Geometry: final body of the model. Coordinates: model frame, mm. A direction names the side the tool comes from. Give positions to 0.01 mm unless a question says otherwise; leave off trailing zeros. Write each loop counter-clockwise with the first axis right and the second up, starting at its lowest first coordinate (ties: lowest second). Pieces come first, ordered by that corner, then holes.
Q1. Cut plane B-B on y = -2.3. Return the cut outline in (x, z), plus the area to 3 significant figures.
Q2. Reachability of faces 5 (the face through (2.848, 0, 12)), 6 (the face through (-2.6, 0.7, 11)) from +Z, -Z, +X, -X, +Y, -Y: full face, straight path, thin tool, end or side. Return the list, or none.
Q3. Pin query (flat end, axial travel): pin 1 (3 mm diameter, centred on x = 0.5, y = 0, fed in from -Z) (3 decimals). Return the tip coordinate at first contact, or that it passes through.
Q4. Draft query along Y for faces 1 (the face through (0, -2.79, 12)), 2 (the face through (0.1, -0.3, 10.9)), 3 (the face through (-1.216, 1.115, 5.306)), 4 (the face through (-0.54, -2.44, 5.42)). Return one class per face: pulls with the +Y half, pulls with the -Y half, needs draft (parallel to the pull), parting line crosses it, or undercut.
Q5. Cut plane A-A on z = 1.75. Return the cut outline in (x, y).
Q6. Line query: L1, parallel to Y at x = 0, z = 6.25; L2, parallel to Y at x = -1.35, z = 7; L3, parallel to Z at x = -2.55, y = 1.05. Output: solid intervals per line, ascending.
```python
from build123d import *

# Parameters (mm, degrees)
SKETCH_1_R                   = 2.5
EXTRUDE_1_DEPTH              = 11
SKETCH_2_W                   = 5.696018396
SKETCH_2_H                   = 5.580245664
EXTRUDE_2_DEPTH              = 2
HOLE_WIZARD_M4_1_D           = 3.3
HOLE_WIZARD_M4_1_DEPTH       = 10.1
HOLE_WIZARD_M4_1_CSINK_D     = 4.05
HOLE_WIZARD_M4_1_CSINK_ANGLE = 90
HOLE_WIZARD_M4_1_TIP         = 0.991420021


with BuildPart() as part:
    # 스케치1 → 보스-돌출1 (new body)
    with BuildSketch(Plane.XY):
        Circle(SKETCH_1_R)
    extrude(amount=EXTRUDE_1_DEPTH)

    # 스케치2 → 보스-돌출2 (add)
    with BuildSketch(Plane.XY.offset(11)):
        Rectangle(SKETCH_2_W, SKETCH_2_H)
    extrude(amount=EXTRUDE_2_DEPTH)

    # M4 나사 구멍1
    with Locations(Plane(origin=(0, 0, 0), x_dir=(-1, 0, 0), z_dir=(0, 0, -1))):
        with Locations((0, 0)):
            CounterSinkHole(HOLE_WIZARD_M4_1_D / 2, HOLE_WIZARD_M4_1_CSINK_D / 2, depth=HOLE_WIZARD_M4_1_DEPTH, counter_sink_angle=HOLE_WIZARD_M4_1_CSINK_ANGLE)
            with Locations((0, 0, -(HOLE_WIZARD_M4_1_DEPTH + HOLE_WIZARD_M4_1_TIP / 2))):  # 118° drill point
                Cone(0, HOLE_WIZARD_M4_1_D / 2, HOLE_WIZARD_M4_1_TIP, mode=Mode.SUBTRACT)


solid = part.part
```
Data:
1. outline: (-2.85, 11) - (-0.98, 11) - (-0.98, 0) - (0.98, 0) - (0.98, 11) - (2.85, 11) - (2.85, 13) - (-2.85, 13) - close
1. area: 32.9 mm2
2. face 5: +Z, -Z, +X, +Y, -Y
2. face 6: -Z
3. pin 1: stops at z = 0.025
4. face 1: pulls with the -Y half
4. face 2: undercut
4. face 3: undercut
4. face 4: parting line crosses it
5. outline: circle Ø5 at (0, 0); hole circle Ø3.3 at (0, 0)
6. L1: y = -2.5 to -1.65, 1.65 to 2.5
6. L2: y = -2.1 to -0.95, 0.95 to 2.1
6. L3: z = 11 to 13
